from build123d import *

# Parameters (mm, degrees)
SKETCH1_R           = 23
SKETCH1_R_2         = 21
BOSS_EXTRUDE1_DEPTH = 12
CUT_EXTRUDE1_START  = 19.798989767
CUT_EXTRUDE1_DEPTH  = 3.113888708
BOSS_EXTRUDE2_START = -1
SKETCH3_R           = 21
SKETCH3_R_2         = 6
BOSS_EXTRUDE2_DEPTH = 1


# Read off the part's stored shape, not the designer's step: Cut-Extrude1
with BuildPart() as part:
    # Sketch1 → Boss-Extrude1 (new body)
    with BuildSketch(Plane(origin=(0, 0, 0), x_dir=(0, 0, -1), z_dir=(1, 0, 0))):
        Circle(SKETCH1_R)
        Circle(SKETCH1_R_2, mode=Mode.SUBTRACT)
    extrude(amount=BOSS_EXTRUDE1_DEPTH)

    # Cut-Extrude1 outline → Cut-Extrude1 (cut)
    with BuildSketch(Plane(origin=(0, 0, 0), x_dir=(1, 0, 0), z_dir=(0, 1, 0)).offset(CUT_EXTRUDE1_START)):
        with BuildLine():
            Line((3.85, 2), (7.15, 2))
            add(Edge.make_bspline(
                [(7.15, 2), (7.817845854, 2), (8.470708827, 2.278069652), (9.392173726, 3.213958296), (9.654566139, 3.870579279), (9.645305955, 5.165184319), (9.383600306, 5.79959696), (8.460809694, 6.727038511), (7.818179406, 7), (7.15, 7)],
                knots=[0, 0, 0, 0, 0.25, 0.25, 0.5, 0.5, 0.75, 0.75, 1, 1, 1, 1], degree=3))
            Line((7.15, 7), (3.85, 7))
            add(Edge.make_bspline(
                [(3.85, 7), (3.181977083, 7), (2.533951966, 6.72160004), (1.622306662, 5.805707302), (1.355260445, 5.166655745), (1.344899993, 3.873398622), (1.601104231, 3.221423625), (2.533655688, 2.273000364), (3.182229779, 2), (3.85, 2)],
                knots=[0, 0, 0, 0, 0.25, 0.25, 0.5, 0.5, 0.75, 0.75, 1, 1, 1, 1], degree=3))
        make_face()
        with BuildLine():
            add(Edge.make_bspline(
                [(7.15, -2), (7.817845854, -2), (8.470708827, -2.278069652), (9.392173726, -3.213958296), (9.654566139, -3.870579279), (9.645305955, -5.165184319), (9.383600306, -5.79959696), (8.460809694, -6.727038511), (7.818179406, -7), (7.15, -7)],
                knots=[0, 0, 0, 0, 0.25, 0.25, 0.5, 0.5, 0.75, 0.75, 1, 1, 1, 1], degree=3))
            Line((7.15, -2), (3.85, -2))
            add(Edge.make_bspline(
                [(3.85, -7), (3.181977083, -7), (2.533951966, -6.72160004), (1.622306662, -5.805707302), (1.355260445, -5.166655745), (1.344899993, -3.873398622), (1.601104231, -3.221423625), (2.533655688, -2.273000364), (3.182229779, -2), (3.85, -2)],
                knots=[0, 0, 0, 0, 0.25, 0.25, 0.5, 0.5, 0.75, 0.75, 1, 1, 1, 1], degree=3))
            Line((3.85, -7), (7.15, -7))
        make_face()
    extrude(amount=CUT_EXTRUDE1_DEPTH, mode=Mode.SUBTRACT)

    # Sketch3 → Boss-Extrude2 (add)
    with BuildSketch(Plane(origin=(12, 0, 0), x_dir=(0, 0, -1), z_dir=(1, 0, 0)).offset(BOSS_EXTRUDE2_START)):
        Circle(SKETCH3_R)
        Circle(SKETCH3_R_2, mode=Mode.SUBTRACT)
    extrude(amount=BOSS_EXTRUDE2_DEPTH)


solid = part.part
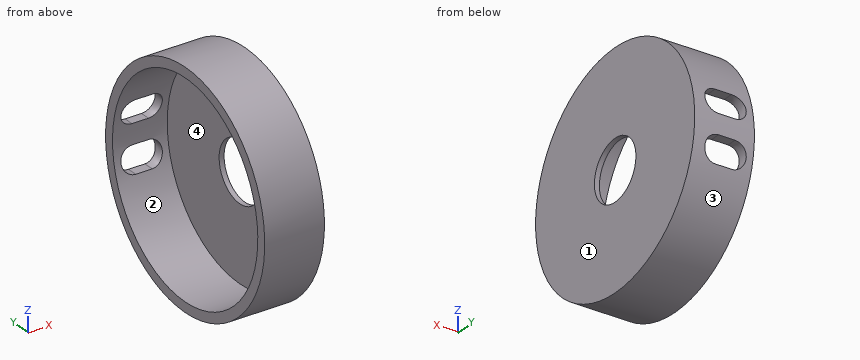
Verification items for the finished model (mm, model axes). Face numbers are marked on the shaded views. Give positions to 0.01 mm unless a question says otherwise; leave off trailing zeros. Order: outer loops, then holes, each group sorted by start corner. A loop starts at its lowest first (then second) coordinate and runs counter-clockwise, first axis right, second up. Notation, with made-up numbers: M -26,77 L 23,77 A22 cw 23,109 Z; hole C 4,-11 d3. An arc over 180 degrees is marked long. Answer as a JSON object with one key per item and string values. Group by question number.
1) Scan lines: line 1 along X through (y, z) = (2.5, -13.5); line 2 along Y through (x, z) = (6.5, 0); line 3 along Y through (x, z) = (5.5, -11). Record each from-to range of solid material in increasing order. Write a range as [from, to].
2) Cross-section at B-B (x = 4.5). Enter the section's corners in (y, z).
3) Cross-section at D-D (z = 14.5). Enter the section's corners in (x, y), then the cut area to 3 significant figures.
4) Cross-section at A-A (z = 0). Enter the section's corners in (x, y).
5) Mould release check, pull along Z, two halves, no side actions. Record for the marked faces 1, 2, 3 and 4: released by +Z, released by -Z, zero draft, split by the parting line, or undercut.
6) Depth check by flat-ended pin: pin 1 Ø1.5 at (y, z) = (0.5, -17) entering from -X; pin 2 Ø6 at (x, z) = (4, -5) entering from -Y; pin 3 Ø2 at (x, z) = (11, -13.5) entering from -Y. Enter the tip coordinate at first touch or a pass-through.
Result sheet:
{
 "1": {"line 1": "x = [11, 12]", "line 2": "y = [-23, -21], [21, 23]", "line 3": "y = [-20.2, -17.89], [17.89, 20.2]"},
 "2": {"outline": "M 19.8,-7 A21 cw long 19.8,7 L 21.91,7 A23 ccw long 21.91,-7 Z; M 20.9,-2 L 22.91,-2 A23 ccw 22.91,2 L 20.9,2 A21 cw Z"},
 "3": {"outline": "M 0,-17.85 L 12,-17.85 L 12,17.85 L 0,17.85 L 0,15.19 L 11,15.19 L 11,-15.19 L 0,-15.19 Z", "area": "94.3 mm2"},
 "4": {"outline": "M 0,-23 L 12,-23 L 12,-6 L 11,-6 L 11,-21 L 0,-21 Z; M 0,21 L 11,21 L 11,6 L 12,6 L 12,23 L 0,23 Z"},
 "5": {"face 1": "zero draft", "face 2": "undercut", "face 3": "split by the parting line", "face 4": "undercut"},
 "6": {"pin 1": "stops at x = 11", "pin 2": "stops at y = -22.91", "pin 3": "stops at y = -19.31"}
}
